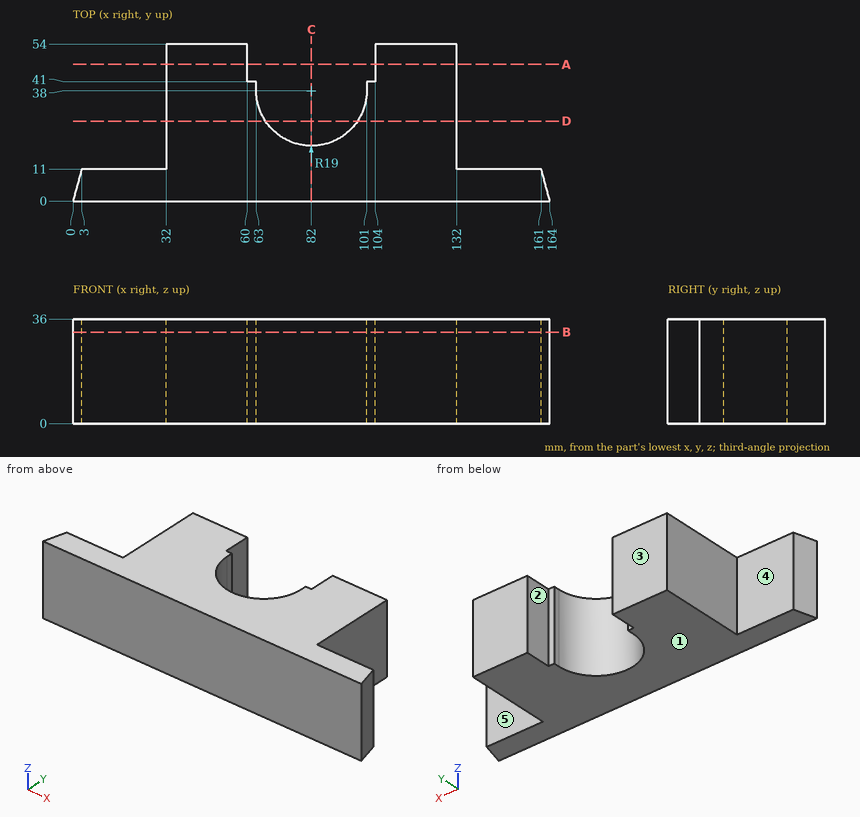
Here's the drawing with two shaded views (mm, measured from the low corner). I have some questions. A direction names the side the tool comes from. Coordinates: 2 decimals unless noted, no trailing zeros. Order: outer loops, then holes, each group sorted by start corner. A loop starts at its lowest first (then second) coordinate and runs counter-clockwise, first axis right, second up. Notation, with made-up numbers: (35, -7.75) -> (68, -7.75) arc R19 cw to (68, 21.25) -> close; hole circle Ø11 at (-19.75, 54.25). An arc over 180 degrees is marked (long way). One line per question, with ' | ' between items.
Q1. I'm going to push flat-ended pins straight in: P1, Ø4, axis at y = 19, z = 29.5, coming from the +X side; P2, Ø0.9, axis at x = 102, z = 19, coming from the +Y side; P3, Ø3, axis at x = 46, z = 10, coming from the -Y side; P4, Ø8, axis at y = 25.5, z = 25, coming from the -X side. Where does each tip first touch, or does it pass through?
Return value:
P1: x = 132 | P2: y = 41 | P3: y = 0 | P4: x = 32
Q2. On a 3-axis mill with a long thin cutter (end or side, diameter ignored), from which of +Z, -Z, +X, -X, +Y, -Y can I reach the whole of each face in a straight line? I mean the marked faces 1, 2, 3, 4 and 5. Say none if no direction works.
Return value:
face 1: -Z, +X, -X, +Y, -Y | face 2: +Z, -Z, +Y | face 3: +Z, -Z, +X, -X, +Y | face 4: +Z, -Z, -X, +Y | face 5: +Z, -Z, +X, +Y
Q3. Imagine slicing it at D-D on y = 27.5. Please give me the cut outline in (x, z), and give its area (3 significant figures).
Return value:
outline: (32, 0) -> (66.16, 0) -> (66.16, 36) -> (32, 36) -> close; (97.84, 0) -> (132, 0) -> (132, 36) -> (97.84, 36) -> close | area: 2,460 mm²
Q4. Imagine slicing it at B-B on z = 31.5. Please give me the cut outline in (x, y), and give its area (3 significant figures).
Return value:
outline: (0, 0) -> (164, 0) -> (161, 11) -> (132, 11) -> (132, 54) -> (104, 54) -> (104, 41) -> (101, 41) -> (101, 38) arc R19 cw to (63, 38) -> (63, 41) -> (60, 41) -> (60, 54) -> (32, 54) -> (32, 11) -> (3, 11) -> close | area: 4,820 mm²
Q5. Imagine slicing it at C-C on x = 82. Please give me the cut outline in (y, z), and give its area (3 significant figures).
Return value:
outline: (0, 0) -> (19, 0) -> (19, 36) -> (0, 36) -> close | area: 684 mm²
Q6. Imagine slicing it at A-A on y = 47. Please give me the cut outline in (x, z), and give its area (3 significant figures).
Return value:
outline: (32, 0) -> (60, 0) -> (60, 36) -> (32, 36) -> close; (104, 0) -> (132, 0) -> (132, 36) -> (104, 36) -> close | area: 2,020 mm²
Q7. If I drill on L1, parallel to X at y = 41.5, z = 17.5; L2, parallel to X at y = 18.5, z = 7.5; L3, parallel to Y at x = 137.5, z = 28, over which ranges is the centre line in solid material (lowest first)?
Return value:
L1: 32 to 60, 104 to 132 | L2: 32 to 132 | L3: 0 to 11
